Solid Edge part; units mm, degrees
sketch "Sketch1" plane through (0, 0, 0) normal (0, -1, 0) x (1, 0, 0)
  line L0 (-10, -36) -> (10, -36)
  line L1 (10, -36) -> (10, 36)
  line L2 (10, 36) -> (-10, 36)
  line L3 (-10, 36) -> (-10, -36)
  dimension "D1" = 10
  dimension "D2" = 10
extrude "Protrusion1" add sketch "Sketch1" along normal blind 10
sketch "Sketch2" plane through (0, 0, 0) normal (0, 1, 0) x (-1, 0, 0)
  circle A0 centre (0, 27) radius 6.025
  circle A1 centre (0, -27) radius 6.025
extrude "Cutout1" cut sketch "Sketch2" against normal through all
fillet "Verrundung_1" radius 10 4 edges at (-10, -5, 36) (10, -5, 36) (-10, -5, -36) (10, -5, -36)
fillet "Verrundung_2" radius 4 3 edges at (-10, 0, 0) (10, 0, 0) (0, 0, 36)
sketch "Sketch3" plane through (10, -7, 0) normal (1, 0, 0) x (0, 0, -1)
  line L0 (-12.5, 4.5) -> (-37.5, 4.5)
  line L1 (-37.5, 4.5) -> (-37.5, 10.5)
  line L2 (-37.5, 10.5) -> (-12.5, 10.5)
  line L3 (-12.5, 10.5) -> (-12.5, 4.5)
  line L4 (12.5, 4.5) -> (37.5, 4.5)
  line L5 (37.5, 4.5) -> (37.5, 10.5)
  line L6 (37.5, 10.5) -> (12.5, 10.5)
  line L7 (12.5, 10.5) -> (12.5, 4.5)
  dimension "D1" = 12.5
  dimension "D2" = 12.5
  dimension "D3" = 37.5
  dimension "D4" = 37.5
extrude "Cutout2" cut sketch "Sketch3" against normal through all
chamfer "Fase_1" distance 1 angle 45 1 edges at (0, -2.5, 20.975)
The listing builds one solid part. Answer for the finished solid, in the listing's coordinates (mm). A direction names the side the tool comes from. Give positions to 0.01 mm unless a question says otherwise; leave off trailing zeros. Loops run counter-clockwise (first coordinate to the right, second up) from the corner with the lowest first, then second, coordinate; pieces in that order, holes last.
Item 1: Find the intervals of material crossed by line 1 along Z through (x, y) = (0, -5.25) (3 decimals); line 2 along Y through (x, z) = (6, 15); line 3 along Z through (x, y) = (1.75, -5), in increasing order.
Derived:
line 1: z = -36 to -33.025, -20.975 to 20.975, 33.025 to 36
line 2: y = -10 to -2.5
line 3: z = -35.85 to -32.77, -21.23 to 21.23, 32.77 to 35.85
Item 2: Determine the mould class of faces 1 (the cylindrical face through (-7.15, -6.98, -32.99)), 2 (the cylindrical face through (7.15, -6.98, 32.99)), 3 (the cylindrical face through (0.784, -6.198, -21.026)) for opening direction Z: +Z half, -Z half, draft (parallel to the pull), parting line (faces both ways), or undercut.
Derived:
face 1: -Z half
face 2: +Z half
face 3: undercut
Item 3: A tool of negligible diameter and unlimited length cuts with its end or side. For faces 4 (the flat face through (0, -1, 12.5)), 5 (the flat face through (0, -1, -12.5)), 6 (the flat face through (0, 0, 0)), from which of +Z, -Z, +X, -X, +Y, -Y can it reach the whole face along a straight path? Write none if from no direction.
Derived:
face 4: +Z, +X, -X, +Y
face 5: -Z, +X, -X, +Y
face 6: +Z, -Z, +X, -X, +Y
Item 4: Each of these flat-tipped pins is pushed along its axis until it touches: pin 1 Ø5 at (x, y) = (0.5, -5.5) entering from -Z; pin 2 Ø1 at (x, y) = (7.5, -3.5) entering from +Z; pin 3 Ø9.5 at (x, z) = (2, -30) entering from +Y; pin 4 Ø0.8 at (x, y) = (2.5, -1.5) entering from +Z. Where does it stop, or does it pass through?
Derived:
pin 1: stops at z = -36
pin 2: stops at z = 33.11
pin 3: stops at y = -2.5
pin 4: stops at z = 12.5
Item 5: A cutting plane is placed at B-B (z = -23). Give the vertices of the cut face in (x, y).
Derived:
outline: (-10, -10) - (-4.51, -10) - (-4.51, -2.5) - (-9.71, -2.5) arc R4 ccw to (-10, -4) - close; (4.51, -10) - (10, -10) - (10, -4) arc R4 ccw to (9.71, -2.5) - (4.51, -2.5) - close
Item 6: A cutting plane is placed at C-C (z = -5.5). Give the vertices of the cut face in (x, y), then the cut area to 3 significant figures.
Derived:
outline: (-10, -10) - (10, -10) - (10, -4) arc R4 ccw to (6, 0) - (-6, 0) arc R4 ccw to (-10, -4) - close
area: 193 mm2
Item 7: A cutting plane is placed at A-A (y = -9). Give the number of separate pieces and of enclosed holes in the cut face, then the cut area to 3 significant figures.
Derived:
separate pieces: 1
enclosed holes: 2
area: 1,130 mm2
